Part model, mm, in its own coordinate system. A direction names the side the tool comes from. Round coordinates to 2 decimals unless told otherwise and drop trailing zeros. Order: outer loops, then holes, each group sorted by start corner. A loop starts at its lowest first (then second) coordinate and runs counter-clockwise, first axis right, second up. Notation, with made-up numbers: M 16,-16.5 L 43,-16.5 A22 cw 43,-0.5 Z; hole C 88,7 d7. An arc over 180 degrees is marked long. One line per question, with ' | ' between items.
from build123d import *

# Parameters (mm, degrees)
SKETCH3_R           = 90
BOSS_EXTRUDE1_DEPTH = 37
CHAMFER1_SIZE       = 4
CHAMFER1_SIZE2      = 4.142121255
SKETCH4_W           = 155
SKETCH4_H           = 40
BOSS_EXTRUDE2_DEPTH = 50


with BuildPart() as part:
    # Sketch3 → Boss-Extrude1 (new body)
    with BuildSketch(Plane.XY):
        Circle(SKETCH3_R)
    extrude(amount=BOSS_EXTRUDE1_DEPTH)

    # Chamfer1
    chamfer1_edges = [part.edges().sort_by_distance(p)[0] for p in [
        (-90, 0, 37),
    ]]
    chamfer1_side = [part.faces().sort_by_distance(p)[0] for p in [
        (-90, 0, 18.5),
    ]]
    chamfer(chamfer1_edges, length=CHAMFER1_SIZE, length2=CHAMFER1_SIZE2, reference=chamfer1_side[0])

    # Sketch4 → Boss-Extrude2 (add)
    with BuildSketch(Plane.XY.offset(37)):
        Rectangle(SKETCH4_W, SKETCH4_H)
    extrude(amount=BOSS_EXTRUDE2_DEPTH)


solid = part.part
1) Saw through at A-A (y = 0). List the corners of the cut face in (x, z), plus the area to 3 significant figures.
The answers:
outline: M -90,0 L 90,0 L 90,33 L 85.86,37 L 77.5,37 L 77.5,87 L -77.5,87 L -77.5,37 L -85.86,37 L -90,33 Z | area: 14,400 mm²
2) Saw through at C-C (z = 67.5). List the corners of the cut face in (x, y), plus the area to 3 significant figures.
The answers:
outline: M -77.5,-20 L 77.5,-20 L 77.5,20 L -77.5,20 Z | area: 6,200 mm²
3) Probe line 1 (Z direction, x = 50, y = 24.5); line 2 (Y direction, x = 27, z = 18.5); line 3 (X direction, y = 16.5, z = 74.5). List the from-to ranges inside material, lowest first. Write a range as [from, to].
The answers:
line 1: z = [0, 37] | line 2: y = [-85.85, 85.85] | line 3: x = [-77.5, 77.5]
4) Saw through at D-D (z = 10). List the corners of the cut face in (x, y).
The answers:
outline: C 0,0 d180
5) Which spindle directions (+Z, -Z, +X, -X, +Y, -Y) get a long thin tool onto all of the face, cutting with end or side? Do faces 1 (the face through (-77.5, 0, 62)), 2 (the face through (-1, 20, 62)), 3 (the face through (77.5, 0, 62)), 4 (the face through (-1, -20, 62)). Say none if no direction does.
The answers:
face 1: +Z, -X, +Y, -Y | face 2: +Z, +X, -X, +Y | face 3: +Z, +X, +Y, -Y | face 4: +Z, +X, -X, -Y
6) Drop flat-ended pins along their axis: pin 1 (12 mm diameter, centred on y = -7, z = 49.5, fed in from -X); pin 2 (8 mm diameter, centred on x = -42.5, y = -59.5, fed in from +Z); pin 3 (4 mm diameter, centred on y = 12.5, z = 58, fed in from +X). Give the stop position or say it passes through.
The answers:
pin 1: stops at x = -77.5 | pin 2: stops at z = 37 | pin 3: stops at x = 77.5
7) Saw through at B-B (x = 0). List the corners of the cut face in (y, z).
The answers:
outline: M -90,0 L 90,0 L 90,33 L 85.86,37 L 20,37 L 20,87 L -20,87 L -20,37 L -85.86,37 L -90,33 Z
